The listing builds one solid part. Answer for the finished solid, in the listing's coordinates (mm). A direction names the side the tool comes from. Give positions to 0.01 mm unless a question says otherwise; leave off trailing zeros. Loops run counter-clockwise (first coordinate to the right, second up) from the corner with the lowest first, then second, coordinate; pieces in that order, holes last. Notation, with made-up numbers: (18.5, 89) - (57.5, 89) arc R18 ccw to (57.5, 99) - close; hole circle Ø4 at (0, -12). An arc over 180 degrees is marked (long way). Answer in a Markdown table with one row per item. Add a question column.
```python
from build123d import *

# Parameters (mm, degrees)
BOSS_EXTRUDE1_DEPTH = 15
SKETCH2_R           = 5.5
CUT_EXTRUDE1_DEPTH  = 30
SKETCH3_R           = 5
CUT_EXTRUDE2_DEPTH  = 30
FILLET1_R           = 10
BOSS_EXTRUDE2_DEPTH = 3
FILLET2_R           = 10


with BuildPart() as part:
    # Sketch1 → Boss-Extrude1 (new body, symmetric)
    with BuildSketch(Plane(origin=(0, 0, 0), x_dir=(0, 0, -1), z_dir=(1, 0, 0))):
        Polygon((-55, 5), (-5, 5), (-5, 60), (0, 60), (0, 0), (-55, 0), align=None)
    extrude(amount=BOSS_EXTRUDE1_DEPTH, both=True)

    # Sketch2 → Cut-Extrude1 (cut)
    with BuildSketch(Plane(origin=(0, 5, 0), x_dir=(1, 0, 0), z_dir=(0, 1, 0))):
        with Locations((0, -30)):
            Circle(SKETCH2_R)
    extrude(amount=-CUT_EXTRUDE1_DEPTH, mode=Mode.SUBTRACT)

    # Sketch3 → Cut-Extrude2 (cut)
    with BuildSketch(Plane.XY.offset(5)):
        with Locations((0, 40)):
            Circle(SKETCH3_R)
    extrude(amount=-CUT_EXTRUDE2_DEPTH, mode=Mode.SUBTRACT)

    # Fillet1
    fillet1_edges = [part.edges().sort_by_distance(p)[0] for p in [
        (15, 60, 2.5),
        (15, 2.5, 55),
        (-15, 60, 2.5),
        (-15, 2.5, 55),
    ]]
    fillet(fillet1_edges, radius=FILLET1_R)

    # Sketch4 → Boss-Extrude2 (add)
    with BuildSketch(Plane.ZY.offset(15)):
        Polygon((30, 5), (5, 30), (5, 5), align=None)
    boss_extrude2 = extrude(amount=-BOSS_EXTRUDE2_DEPTH)

    # Mirror1: Boss-Extrude2 across plane
    add(boss_extrude2.mirror(Plane(origin=(0, 0, 0), x_dir=(0, 0, 1), z_dir=(1, 0, 0))))

    # Fillet2
    fillet2_edges = [part.edges().sort_by_distance(p)[0] for p in [
        (0, 5, 5),
    ]]
    fillet(fillet2_edges, radius=FILLET2_R)


solid = part.part
```
(1) Given pin 1 Ø6 at (x, z) = (10.5, 21.5) entering from +Y; pin 2 Ø15 at (x, z) = (-5.5, 43) entering from +Y; pin 3 Ø10 at (x, y) = (-8, 12.5) entering from +Z, each flat-ended and moving along its own axis, determine where each tip first touches the part or whether it passes through.
(2) A cutting plane is placed at A-A on y = 40. Determine the outline of the cut face in (x, z), plus the area to 3 significant figures.
(3) A cutting plane is placed at C-C on z = 20. Determine the outline of the cut face in (x, y), plus the area to 3 significant figures.
(4) The mould has two halves that part along Z. Classify faces 3 (the face through (0, 30, 0)), 4 (the face through (0, 5, 40)), 5 (the face through (11.99, 2.54, 52.15)), 6 (the face through (-0.716, 2.535, 24.547)): pulls with the +Z half, pulls with the -Z half, needs draft (parallel to the pull), parting line crosses it, or undercut.
(5) A cutting plane is placed at D-D on y = 22. Determine the outline of the cut face in (x, z), plus the area to 3 significant figures.
(6) Find the intervals of material crossed by line 1 along Z through (x, y) = (0, 3); line 2 along Y through (x, z) = (0, 1.15); line 3 along X through (y, z) = (2, 30), in increasing order. Write a range as [from, to].
(7) A cutting plane is placed at B-B on x = 0. Determine the outline of the cut face in (y, z), plus the area to 3 significant figures.
(8) A tool of negligible diameter and unlimited length cuts with its end or side. For faces 1 (the face through (0, 0, 21)), 2 (the face through (-0.17, 7.85, 8.01)), from which of +Z, -Z, +X, -X, +Y, -Y can it reach the whole face along a straight path? Write none if from no direction.
Evaluation:
| question | item | result |
|---|---|---|
| 1 | pin 1 | stops at y = 16.1 |
| 1 | pin 2 | stops at y = 5 |
| 1 | pin 3 | stops at z = 25.5 |
| 2 | outline | (-15, 0) - (-5, 0) - (-5, 5) - (-15, 5) - close; (5, 0) - (15, 0) - (15, 5) - (5, 5) - close |
| 2 | area | 100 mm² |
| 3 | outline | (-15, 0) - (15, 0) - (15, 15) - (12, 15) - (12, 5) - (-12, 5) - (-12, 15) - (-15, 15) - close |
| 3 | area | 210 mm² |
| 4 | face 3 | pulls with the -Z half |
| 4 | face 4 | needs draft |
| 4 | face 5 | pulls with the +Z half |
| 4 | face 6 | undercut |
| 5 | outline | (-15, 0) - (15, 0) - (15, 13) - (12, 13) - (12, 5) - (-12, 5) - (-12, 13) - (-15, 13) - close |
| 5 | area | 198 mm² |
| 6 | line 1 | z = [0, 24.5], [35.5, 55] |
| 6 | line 2 | y = [0, 35], [45, 60] |
| 6 | line 3 | x = [-15, -5.5], [5.5, 15] |
| 7 | outline | (0, 0) - (35, 0) - (35, 5) - (15, 5) arc R10 cw to (5, 15) - (5, 24.5) - (0, 24.5) - close; (0, 35.5) - (5, 35.5) - (5, 55) - (0, 55) - close; (45, 0) - (60, 0) - (60, 5) - (45, 5) - close |
| 7 | area | 466 mm² |
| 8 | face 1 | +Z, -Z, +X, -X, -Y |
| 8 | face 2 | +Z, +Y |
